Design review of the part built by this model. Coordinates are the model's own, in mm. Round coordinates to 2 decimals unless told otherwise and drop trailing zeros. Order: outer loops, then holes, each group sorted by start corner. A loop starts at its lowest first (then second) coordinate and runs counter-clockwise, first axis right, second up. Notation, with made-up numbers: M 80.5,64 L 125.5,64 A21 cw 125.5,68 Z; hole C 72.5,88 d5. An arc over 180 degrees is marked long. Use a Markdown table: item, result. Add a question column.
(1) To check wall thickness, follow probe 1 along X at (y, z) = (6, 0); probe 2 along Z at (x, y) = (8, -0.25); probe 3 along Z at (x, y) = (75, -4). State the ranges of each line that lie inside material, in increasing order. Write a range as from..to.
(2) For pin 1 (1 mm diameter, centred on x = 92, y = 8.5, fed in from +Z); pin 2 (6 mm diameter, centred on x = 247.5, y = -4.5, fed in from +Z); pin 3 (6 mm diameter, centred on x = 98.5, y = -8.5, fed in from -Z), all flat-tipped, find the tip position at first contact; note any pin that passes through.
(3) Take a section at B-B (x = -27). Write out the cut boundary in (y, z).
(4) Take a section at D-D (x = 225.5). Write out the cut boundary in (y, z).
(5) Take a section at C-C (y = 6). Count the separate pieces of the cut face and the enclosed holes in it, then the cut area to 3 significant figures.
(6) Take a section at A-A (z = -145). Write out the cut boundary in (x, y).
(7) The part is to be moulded in two halves that separate along X. For faces 1 (the face through (-307.51, 0.18, -68.29)), 2 (the face through (74, -12.5, 206)), 3 (the face through (-212.328, -0.175, -47.15)), say which applies: released by +X, released by -X, zero draft, split by the parting line, or undercut.
```python
from build123d import *

# Parameters (mm, degrees)
SKETCH1_R           = 315
SKETCH1_R_2         = 217.5
SKETCH1_R_3         = 6
BOSS_EXTRUDE1_DEPTH = 12.5


with BuildPart() as part:
    # Sketch1 → Boss-Extrude1 (new, symmetric)
    with BuildSketch(Plane(origin=(0, 0, 0), x_dir=(1, 0, 0), z_dir=(0, 1, 0))):
        with Locations(Location((0, 0, 0), (0, 0, 270))):
            Circle(SKETCH1_R)
        with Locations(Location((0, 0, 0), (0, 0, 270))):
            Circle(SKETCH1_R_2, mode=Mode.SUBTRACT)
        with Locations(Location((0, 240, 0), (0, 0, 270))):
            Circle(SKETCH1_R_3, mode=Mode.SUBTRACT)
        with Locations(Location((169.705627485, 169.705627485, 0), (0, 0, 270))):
            Circle(SKETCH1_R_3, mode=Mode.SUBTRACT)
        with Locations(Location((240, 0, 0), (0, 0, 270))):
            Circle(SKETCH1_R_3, mode=Mode.SUBTRACT)
        with Locations(Location((169.705627485, -169.705627485, 0), (0, 0, 270))):
            Circle(SKETCH1_R_3, mode=Mode.SUBTRACT)
        with Locations(Location((0, -240, 0), (0, 0, 270))):
            Circle(SKETCH1_R_3, mode=Mode.SUBTRACT)
        with Locations(Location((-169.705627485, -169.705627485, 0), (0, 0, 270))):
            Circle(SKETCH1_R_3, mode=Mode.SUBTRACT)
        with Locations(Location((-240, 0, 0), (0, 0, 270))):
            Circle(SKETCH1_R_3, mode=Mode.SUBTRACT)
        with Locations(Location((-169.705627485, 169.705627485, 0), (0, 0, 270))):
            Circle(SKETCH1_R_3, mode=Mode.SUBTRACT)
    extrude(amount=BOSS_EXTRUDE1_DEPTH, both=True)


solid = part.part
```
Verdict:
| question | item | result |
|---|---|---|
| 1 | probe 1 | x = -315..-246, -234..-217.5, 217.5..234, 246..315 |
| 1 | probe 2 | z = -314.9..-217.35, 217.35..314.9 |
| 1 | probe 3 | z = -305.94..-204.16, 204.16..305.94 |
| 2 | pin 1 | stops at z = 301.42 |
| 2 | pin 2 | stops at z = 198.61 |
| 2 | pin 3 | stops at z = -300.17 |
| 3 | outline | M -12.5,-313.84 L 12.5,-313.84 L 12.5,-215.82 L -12.5,-215.82 Z; M -12.5,215.82 L 12.5,215.82 L 12.5,313.84 L -12.5,313.84 Z |
| 4 | outline | M -12.5,-219.94 L 12.5,-219.94 L 12.5,219.94 L -12.5,219.94 Z |
| 5 | separate pieces | 1 |
| 5 | enclosed holes | 9 |
| 5 | area | 162,000 mm^2 |
| 6 | outline | M -279.64,-12.5 L -162.11,-12.5 L -162.11,12.5 L -279.64,12.5 Z; M 162.11,-12.5 L 279.64,-12.5 L 279.64,12.5 L 162.11,12.5 Z |
| 7 | face 1 | split by the parting line |
| 7 | face 2 | zero draft |
| 7 | face 3 | undercut |
